Autodesk Inventor part; units mm, degrees
ref_plane "Work Plane1" through (39.3, 0, 21.15) normal (0, 0, -1) x (-1, 0, 0)
ref_plane "YZ Plane" through (0, 0, 0) normal (1, 0, 0) x (0, 1, 0)
ref_plane "XZ Plane" through (0, 0, 0) normal (0, 1, 0) x (-1, 0, 0)
sketch "Sketch1" plane through (0, 0, 0) normal (0, 1, 0) x (-1, 0, 0)
  line L0 (0, 0) -> (-42.3, 0)
  line L1 (-42.3, 0) -> (-42.3, 42.3)
  line L2 (-42.3, 42.3) -> (0, 42.3)
  line L3 (0, 42.3) -> (0, 0)
  dimension "d0" = 42.3
  dimension "d1" = 42.3
extrude "Extrusion1" add sketch "Sketch1" along normal blind 10
chamfer "Chamfer1" distance 3 angle 45 4 edges at (42.3, 5, 42.3) (0, 5, 42.3) (0, 5, 0) (42.3, 5, 0)
sketch "Sketch2" plane through (0, 10, 0) normal (0, 1, 0) x (1, 0, 0)
  line L0 (0.15, -42.15) -> (42.15, -42.15)
  line L1 (42.15, -42.15) -> (42.15, -0.15)
  line L2 (42.15, -0.15) -> (0.15, -0.15)
  line L3 (0.15, -0.15) -> (0.15, -42.15)
  line L4 (0.15, -42.15) -> (42.15, -0.15) construction
  line L5 (42.15, -42.15) -> (0.15, -0.15) construction
  point P0 (0, 0)
  point P1 (21.15, -21.15)
  dimension "d7" = 42
  dimension "d8" = 42
extrude "Extrusion2" add sketch "Sketch2" along normal blind 14
fillet "Fillet1" radius 6 4 edges at (42.15, 17, 42.15) (42.15, 17, 0.15) (0.15, 17, 42.15) (0.15, 17, 0.15)
sketch "Sketch3" plane through (0, 24, 0) normal (0, 1, 0) x (1, 0, 0)
  line L0 (0, -42.3) -> (42.3, -42.3)
  line L1 (42.3, -42.3) -> (42.3, 0)
  line L2 (42.3, 0) -> (0, 0)
  line L3 (0, 0) -> (0, -42.3)
  line L4 (0, -42.3) -> (42.3, 0) construction
  line L5 (42.3, -42.3) -> (0, 0) construction
  point P0 (0, 0)
  point P1 (21.15, -21.15)
  dimension "d12" = 42.3
  dimension "d13" = 42.3
extrude "Extrusion3" add sketch "Sketch3" along normal blind 10
chamfer "Chamfer2" distance 3 angle 45 4 edges at (42.3, 29, 42.3) (42.3, 29, 0) (0, 29, 0) (0, 29, 42.3)
ref_plane "Work Plane1" through (39.3, 0, 21.15) normal (0, 0, -1) x (-1, 0, 0)
sketch "Sketch4" plane through (0, 34, 0) normal (0, 1, 0) x (1, 0, 0)
  circle A0 centre (21.15, -21.15) radius 11
  point P0 (0, 0)
  dimension "d19" = 22
extrude "Extrusion4" add sketch "Sketch4" along normal blind 2.03
sketch "Sketch5" plane through (21.15, 36.03, 21.15) normal (0, 1, 0) x (1, 0, 0)
  circle A0 centre (0, 0) radius 11
  circle A1 centre (0, 0) radius 2.26
  point P0 (-21.15, 21.15)
  dimension "d22" = 4.52
extrude "Extrusion5" add sketch "Sketch5" along normal blind 14 contours A1
sketch "Sketch6" plane through (0, 34, 0) normal (0, 1, 0) x (1, 0, 0)
  circle A0 centre (21.15, -21.15) radius 11
  line L0 (5.655, -36.645) -> (36.645, -5.655) construction
  line L1 (36.645, -36.645) -> (5.655, -5.655) construction
  circle A1 centre (5.655, -5.655) radius 1.5
  circle A2 centre (36.645, -5.655) radius 1.5
  circle A3 centre (36.645, -36.645) radius 1.5
  circle A4 centre (5.655, -36.645) radius 1.5
  point P0 (0, 0)
  dimension "d25" = 30.99
  dimension "d26" = 30.99
  dimension "d27" = 3
  dimension "d28" = 3
  dimension "d29" = 3
  dimension "d30" = 3
extrude "Extrusion6" cut sketch "Sketch6" against normal blind 4.5 contours A1 | A2 | A3 | A4
thread "Thread1"
thread "Thread2"
thread "Thread3"
thread "Thread4"
sketch "Sketch7" plane through (0, 0, 0) normal (0, -1, 0) x (1, 0, 0)
  circle A0 centre (21.15, 21.15) radius 2.25
  point P0 (0, 0)
  dimension "d41" = 4.5
extrude "Extrusion7" add sketch "Sketch7" along normal blind 1
sketch "Sketch8" plane through (0, 0, 0) normal (0, -1, 0) x (1, 0, 0)
  line L0 (5.65, 5.65) -> (36.65, 36.65) construction
  line L1 (36.65, 5.65) -> (5.65, 36.65) construction
  circle A0 centre (5.65, 36.65) radius 1.5
  circle A1 centre (36.65, 36.65) radius 1.5
  circle A2 centre (36.65, 5.65) radius 1.5
  circle A3 centre (5.65, 5.65) radius 1.5
  point P0 (0, 0)
  point P1 (21.15, 21.15)
  dimension "d44" = 31
  dimension "d45" = 31
  dimension "d46" = 3
  dimension "d47" = 3
  dimension "d48" = 3
  dimension "d49" = 3
extrude "Extrusion8" cut sketch "Sketch8" against normal blind 0.5
properties part number "NEMA17"
Build history of the part. All positions in model axes, mm. A direction names the side the tool comes from. Coordinates: 2 decimals unless noted, no trailing zeros. Write each loop counter-clockwise with the first axis right and the second up, starting at its lowest first coordinate (ties: lowest second). Pieces come first, ordered by that corner, then holes.
(1) Mould opens along X. For faces 1 (the flat face through (40.8, 4.9, 40.8)), 2 (the flat face through (21, 17, 42.15)), 3 (the flat face through (0.15, 17, 21)), 4 (the cylindrical face through (35.146, 31.782, 5.589)) say: pulls with the +X half, pulls with the -X half, needs draft (parallel to the pull), parting line crosses it, or undercut.
(2) Pin check, flat tips, straight feed: pin 1 Ø3 at (x, z) = (32.5, 14) entering from -Y; pin 2 Ø10 at (y, z) = (44, 22) entering from +X; pin 3 Ø6 at (x, y) = (6.5, 35.5) entering from +Z; pin 4 Ø3.5 at (x, z) = (5.655, 36.645) entering from +Y. Stop position of each tip, or through.
(3) Drill centre lines: line 1 (Z direction, x = 36.65, y = 0.2); line 2 (Y direction, x = 25, z = 11); line 3 (X direction, y = 12, z = 31). Where is each one in solid material? Low to high.
(4) Cut at D-D on z = 21.15. List the corners of the cut face in (x, y).
(5) Cut at A-A on x = 8. List the corners of the cut face in (y, z).
(6) Cut at B-B on z = 9.5. List the corners of the cut face in (x, y), and give its area (3 significant figures).
(7) 3-axis set-ups, long thin cutter, end or side, ignore diameter. For faces 5 (the flat face through (6, 29.5, 37)), 6 (the flat face through (37, 0.5, 37)), 7 (the flat face through (21, 17, 0.15)): which of +Z, -Z, +X, -X, +Y, -Y reach the whole face in a straight line?
(8) Cut at C-C on x = 17. List the corners of the cut face in (y, z), and give its area (3 significant figures).
Working result:
1. face 1: pulls with the +X half
1. face 2: needs draft
1. face 3: pulls with the -X half
1. face 4: undercut
2. pin 1: stops at y = 0
2. pin 2: stops at x = 23.41
2. pin 3: stops at z = 42.3
2. pin 4: stops at y = 34
3. line 1: z = 0 to 4.15, 7.15 to 35.15, 38.15 to 42.3
3. line 2: y = 0 to 36.03
3. line 3: x = 0.15 to 42.15
4. outline: (0, 0) - (18.9, 0) - (18.9, -1) - (23.4, -1) - (23.4, 0) - (42.3, 0) - (42.3, 10) - (42.15, 10) - (42.15, 24) - (42.3, 24) - (42.3, 34) - (32.15, 34) - (32.15, 36.03) - (23.41, 36.03) - (23.41, 50.03) - (18.89, 50.03) - (18.89, 36.03) - (10.15, 36.03) - (10.15, 34) - (0, 34) - (0, 24) - (0.15, 24) - (0.15, 10) - (0, 10) - close
5. outline: (0, 0) - (10, 0) - (10, 0.15) - (24, 0.15) - (24, 0) - (34, 0) - (34, 42.3) - (24, 42.3) - (24, 42.15) - (10, 42.15) - (10, 42.3) - (0, 42.3) - close
6. outline: (0, 0) - (42.3, 0) - (42.3, 10) - (42.15, 10) - (42.15, 24) - (42.3, 24) - (42.3, 34) - (0, 34) - (0, 24) - (0.15, 24) - (0.15, 10) - (0, 10) - close
6. area: 1,430 mm2
7. face 5: +Y
7. face 6: -Y
7. face 7: -Z, +X, -X
8. outline: (0, 0) - (10, 0) - (10, 0.15) - (24, 0.15) - (24, 0) - (34, 0) - (34, 10.96) - (36.03, 10.96) - (36.03, 31.34) - (34, 31.34) - (34, 42.3) - (24, 42.3) - (24, 42.15) - (10, 42.15) - (10, 42.3) - (0, 42.3) - close
8. area: 1,480 mm2
